```python
from build123d import *

# Parameters (mm, degrees)
F0_R     = 7
F1_DEPTH = 6.35
F2_DEPTH = 203.2
F3_R     = 4.5
F4_DEPTH = 6.351
F3_R_2   = 2.75
F3_R_3   = 30
F5_DEPTH = 6.351
F7_DEPTH = 6.35


with BuildPart() as f1:
    # F0 (on Top) → F1 (new body)
    with BuildSketch(Plane.XY):
        with BuildLine():
            Line((-82.55, -101.6), (95.25, -101.6))
            Line((95.25, -101.6), (95.25, 101.6))
            Line((95.25, 101.6), (-82.55, 101.6))
            ThreePointArc((-82.55, 101.6), (-87.0401280605, 99.7401280605), (-88.9, 95.25))
            Line((-88.9, 95.25), (-88.9, -95.25))
            ThreePointArc((-88.9, -95.25), (-87.0401280605, -99.7401280605), (-82.55, -101.6))
        make_face()
        Circle(F0_R, mode=Mode.SUBTRACT)
    extrude(amount=F1_DEPTH)

    # F0 (on Top) → F2 (join)
    with BuildSketch(Plane.XY):
        with BuildLine():
            Line((-88.9, -107.95), (95.25, -107.95))
            Line((95.25, -107.95), (95.25, -101.6))
            Line((95.25, -101.6), (-82.55, -101.6))
            ThreePointArc((-82.55, -101.6), (-87.0401280605, -99.7401280605), (-88.9, -95.25))
            Line((-88.9, -95.25), (-88.9, 95.25))
            ThreePointArc((-88.9, 95.25), (-87.0401280605, 99.7401280605), (-82.55, 101.6))
            Line((-82.55, 101.6), (95.25, 101.6))
            Line((95.25, 101.6), (95.25, 107.95))
            Line((95.25, 107.95), (-88.9, 107.95))
            ThreePointArc((-88.9, 107.95), (-93.3901280605, 106.0901280605), (-95.25, 101.6))
            Line((-95.25, 101.6), (-95.25, -101.6))
            ThreePointArc((-95.25, -101.6), (-93.3901280605, -106.0901280605), (-88.9, -107.95))
        make_face()
    extrude(amount=F2_DEPTH)

    # F3 (on face) → F4 (cut, through all)
    with BuildSketch(Plane.YZ.offset(-88.9)):
        with Locations((60.8142944519, 40.7813113481)):
            Circle(F3_R)
        with Locations((32.9124589905, 22.1379009341)):
            Circle(F3_R)
        with Locations((0, 15.5912058)):
            Circle(F3_R)
        with Locations((-32.9124589905, 22.1379009341)):
            Circle(F3_R)
        with Locations((-79.4577048659, 68.6831468095)):
            Circle(F3_R)
        with Locations((-86.0044, 101.5956058)):
            Circle(F3_R)
        with Locations((-79.4577048659, 134.5080647905)):
            Circle(F3_R)
        with Locations((-60.8142944519, 162.4099002519)):
            Circle(F3_R)
        with Locations((-32.9124589905, 181.0533106659)):
            Circle(F3_R)
        with Locations((0, 187.6000058)):
            Circle(F3_R)
        with Locations((32.9124589905, 181.0533106659)):
            Circle(F3_R)
        with Locations((60.8142944519, 162.4099002519)):
            Circle(F3_R)
        with Locations((79.4577048659, 134.5080647905)):
            Circle(F3_R)
        with Locations((86.0044, 101.5956058)):
            Circle(F3_R)
        with Locations((79.4577048659, 68.6831468095)):
            Circle(F3_R)
    extrude(amount=-F4_DEPTH, mode=Mode.SUBTRACT)

    # F3 (on face) → F5 (cut, through all)
    with BuildSketch(Plane.YZ.offset(-88.9)):
        with Locations((-60.8142944519, 40.7813113481)):
            Circle(F3_R)
        with Locations((-34.8, 66.8)):
            Circle(F3_R_2)
        with Locations((34.8, 66.8)):
            Circle(F3_R_2)
        with Locations((34.8, 136.4)):
            Circle(F3_R_2)
        with Locations((-34.8, 136.4)):
            Circle(F3_R_2)
        with Locations((0, 101.6)):
            Circle(F3_R_3)
    extrude(amount=-F5_DEPTH, mode=Mode.SUBTRACT)

    # F6 (on face) → F7 (join)
    with BuildSketch(Plane.XY.offset(203.2)):
        with BuildLine():
            Line((95.25, -101.6), (95.25, 101.6))
            Line((95.25, 101.6), (-82.55, 101.6))
            ThreePointArc((-82.55, 101.6), (-87.0401280605, 99.7401280605), (-88.9, 95.25))
            Line((-88.9, 95.25), (-88.9, -95.25))
            ThreePointArc((-88.9, -95.25), (-87.0401280605, -99.7401280605), (-82.55, -101.6))
            Line((-82.55, -101.6), (95.25, -101.6))
        make_face()
        with BuildLine():
            Line((95.25, 107.95), (-88.9, 107.95))
            ThreePointArc((-88.9, 107.95), (-93.3901280605, 106.0901280605), (-95.25, 101.6))
            Line((-95.25, 101.6), (-95.25, -101.6))
            ThreePointArc((-95.25, -101.6), (-93.3901280605, -106.0901280605), (-88.9, -107.95))
            Line((-88.9, -107.95), (95.25, -107.95))
            Line((95.25, -107.95), (95.25, -101.6))
            Line((95.25, -101.6), (-82.55, -101.6))
            ThreePointArc((-82.55, -101.6), (-87.0401280605, -99.7401280605), (-88.9, -95.25))
            Line((-88.9, -95.25), (-88.9, 95.25))
            ThreePointArc((-88.9, 95.25), (-87.0401280605, 99.7401280605), (-82.55, 101.6))
            Line((-82.55, 101.6), (95.25, 101.6))
            Line((95.25, 101.6), (95.25, 107.95))
        make_face()
    extrude(amount=F7_DEPTH)


solid = f1.part
```
Here's how the part is built. I have some questions about the finished solid (model axes, mm). A direction names the side the tool comes from. Round coordinates to 2 decimals unless told otherwise and drop trailing zeros. Loops run counter-clockwise (first coordinate to the right, second up) from the corner with the lowest first, then second, coordinate; pieces in that order, holes last.
1. If I drill on probe 1 along Z at (x, y) = (-90, 0); probe 2 along Z at (x, y) = (62, 17.5); probe 3 along Y at (x, z) = (-77, 18), over which ranges is the centre line in solid material (lowest first)?
Answers:
probe 1: z = 0 to 11.09, 20.09 to 71.6, 131.6 to 183.1, 192.1 to 209.55
probe 2: z = 0 to 6.35, 203.2 to 209.55
probe 3: y = -107.95 to -101.6, 101.6 to 107.95
2. Thinking about a two-plate mould opening in Z: for faces 3 (the face through (-92.031, -83.953, 68.881)), 4 (the face through (6.466, -2.681, 3.131)), which applies, released by +Z, released by -Z, zero draft, split by the parting line, or undercut?
Answers:
face 3: undercut
face 4: zero draft
3. Suppose I cut it at C-C, the plane y = -60. Please give me the cut outline in (x, z), and give its area (3 significant figures).
Answers:
outline: (-95.25, 0) - (95.25, 0) - (95.25, 6.35) - (-88.9, 6.35) - (-88.9, 36.36) - (-95.25, 36.36) - close; (-95.25, 45.21) - (-88.9, 45.21) - (-88.9, 157.98) - (-95.25, 157.98) - close; (-95.25, 166.84) - (-88.9, 166.84) - (-88.9, 203.2) - (95.25, 203.2) - (95.25, 209.55) - (-95.25, 209.55) - close
area: 3,560 mm2
4. For faces 1 (the face through (-92.031, -35.158, 139.127)), 2 (the face through (-88.9, -23, 125)), which set-ups out of +Z, -Z, +X, -X, +Y, -Y let a thin tool reach every point of the face, with its end or its side?
Answers:
face 1: +X, -X
face 2: +X
5. Suppose I cut it at A-A, the plane y = 0. Please give me the cut outline in (x, z), and give its area (3 significant figures).
Answers:
outline: (-95.25, 0) - (-7, 0) - (-7, 6.35) - (-88.9, 6.35) - (-88.9, 11.09) - (-95.25, 11.09) - close; (-95.25, 20.09) - (-88.9, 20.09) - (-88.9, 71.6) - (-95.25, 71.6) - close; (-95.25, 131.6) - (-88.9, 131.6) - (-88.9, 183.1) - (-95.25, 183.1) - close; (-95.25, 192.1) - (-88.9, 192.1) - (-88.9, 203.2) - (95.25, 203.2) - (95.25, 209.55) - (-95.25, 209.55) - close; (7, 0) - (95.25, 0) - (95.25, 6.35) - (7, 6.35) - close
area: 3,090 mm2
6. Will these pins go through, and if not, where does the flat tip stop? pin 1 (4 mm diameter, centred on y = -5.5, z = 154.5, fed in from +X); pin 2 (5 mm diameter, centred on y = 34.8, z = 66.8, fed in from -X).
Answers:
pin 1: stops at x = -88.9
pin 2: passes through
7. Suppose I cut it at D-D, the plane z = 145.5. Please give me the cut outline in (x, y), and give its area (3 significant figures).
Answers:
outline: (-95.25, -101.6) arc R6.35 ccw to (-88.9, -107.95) - (95.25, -107.95) - (95.25, -101.6) - (-82.55, -101.6) arc R6.35 cw to (-88.9, -95.25) - (-88.9, 95.25) arc R6.35 cw to (-82.55, 101.6) - (95.25, 101.6) - (95.25, 107.95) - (-88.9, 107.95) arc R6.35 ccw to (-95.25, 101.6) - close
area: 3,710 mm2
8. Suppose I cut it at B-B, the plane x = -54.5. Please give me the cut outline in (y, z), and give its area (3 significant figures).
Answers:
outline: (-107.95, 0) - (107.95, 0) - (107.95, 209.55) - (-107.95, 209.55) - close; hole (-101.6, 6.35) - (101.6, 6.35) - (101.6, 203.2) - (-101.6, 203.2) - close
area: 5,240 mm2
